Build history of the part. All positions in model axes, mm. A direction names the side the tool comes from. Give positions to 0.01 mm unless a question says otherwise; leave off trailing zeros. Loops run counter-clockwise (first coordinate to the right, second up) from the corner with the lowest first, then second, coordinate; pieces in that order, holes last. Notation, with made-up numbers: (-36.5, 19) -> (21.5, 19) arc R31 ccw to (21.5, 43) -> close; hole circle Ø9 at (-3.5, 47.5). An arc over 180 degrees is marked (long way). Answer in a Markdown table with one row per item. Add a question column.
from build123d import *

# Parameters (mm, degrees)
F2_DEPTH = 2.2225
F3_DEPTH = 12.7
F4_T     = -2.54


with BuildPart() as f2:
    # F0 (on Front) → F2 (new body, symmetric)
    with BuildSketch(Plane.XZ):
        with BuildLine():
            Line((40.6019, 72.8091), (-40.6019, 72.8091))
            ThreePointArc((-40.6019, 72.8091), (-43.295977, 71.693177), (-44.4119, 68.9991))
            Line((-44.4119, 68.9991), (-44.4119, -68.9991))
            ThreePointArc((-44.4119, -68.9991), (-43.295977, -71.693177), (-40.6019, -72.8091))
            Line((-40.6019, -72.8091), (40.6019, -72.8091))
            ThreePointArc((40.6019, -72.8091), (43.295977, -71.693177), (44.4119, -68.9991))
            Line((44.4119, -68.9991), (44.4119, 68.9991))
            ThreePointArc((44.4119, 68.9991), (43.295977, 71.693177), (40.6019, 72.8091))
        make_face()
    extrude(amount=F2_DEPTH, both=True)

    # F1 (on face) → F3 (cut, symmetric)
    with BuildSketch(Plane.XZ):
        with BuildLine():
            Line((15.494, -23.90966), (-15.494, -23.90966))
            ThreePointArc((-15.494, -23.90966), (-17.739064, -24.839596), (-18.669, -27.08466))
            Line((-18.669, -27.08466), (-18.669, -58.07266))
            ThreePointArc((-18.669, -58.07266), (-17.739064, -60.317724), (-15.494, -61.24766))
            Line((-15.494, -61.24766), (15.494, -61.24766))
            ThreePointArc((15.494, -61.24766), (17.739064, -60.317724), (18.669, -58.07266))
            Line((18.669, -58.07266), (18.669, -27.08466))
            ThreePointArc((18.669, -27.08466), (17.739064, -24.839596), (15.494, -23.90966))
        make_face()
    extrude(amount=F3_DEPTH, both=True, mode=Mode.SUBTRACT)

    # F4
    f4_openings = [f2.faces().sort_by_distance(p)[0] for p in [
        (0, 2.2225, 5.113505),
    ]]
    offset(amount=F4_T, openings=f4_openings)


solid = f2.part
(1) Saw through at B-B, the plane z = -40.5. List the corners of the cut face in (x, y), then the cut area to 3 significant figures.
(2) 3-axis set-ups, long thin cutter, end or side, ignore diameter. For faces 4 (the flat face through (-1, 0.317, 17)), 5 (the flat face through (18.669, 0, -43)), 6 (the cylindrical face through (-43.33, -0.03, -71.66)): which of +Z, -Z, +X, -X, +Y, -Y reach the whole face in a straight line?
(3) Saw through at C-C, the plane y = -1.55. List the corners of the cut face in (x, z) (3 decimals), then the cut area to 3 significant figures.
(4) Wall check: line 1 along Z through (x, y) = (3, 2); line 2 along X through (y, z) = (1.5, -64); line 3 along Z through (x, y) = (25.5, 1.2). Give the ranges that are in metal, low to high. Write a range as from..to.
(5) Flat gauge pin, fed straight in: pin 1 Ø3 at (x, z) = (23, -43.5) entering from +Y. Where does the tip first touch, or does it go through?
(6) Saw through at D-D, the plane x = -26. List the corners of the cut face in (y, z), then the cut area to 3 significant figures.
(7) Two-plate mould, pull along X, no slides. Class faces 1 (the cylindrical face through (-17.764, -0.031, -60.293)), 2 (the flat face through (-19, 2.222, -42)), 3 (the flat face through (-44.412, 0, 1)): released by +X, released by -X, zero draft, split by the parting line, or undercut.
(8) Saw through at A-A, the plane x = 13.5. List the corners of the cut face in (y, z).
Worked answers:
| question | item | result |
|---|---|---|
| 1 | outline | (-44.41, -2.22) -> (-18.67, -2.22) -> (-18.67, 2.22) -> (-21.21, 2.22) -> (-21.21, 0.32) -> (-41.87, 0.32) -> (-41.87, 2.22) -> (-44.41, 2.22) -> close; (18.67, -2.22) -> (44.41, -2.22) -> (44.41, 2.22) -> (41.87, 2.22) -> (41.87, 0.32) -> (21.21, 0.32) -> (21.21, 2.22) -> (18.67, 2.22) -> close |
| 1 | area | 150 mm^2 |
| 2 | face 4 | +Y |
| 2 | face 5 | +Y, -Y |
| 2 | face 6 | -Z, -X, +Y, -Y |
| 3 | outline | (-44.412, -68.999) arc R3.81 ccw to (-40.602, -72.809) -> (40.602, -72.809) arc R3.81 ccw to (44.412, -68.999) -> (44.412, 68.999) arc R3.81 ccw to (40.602, 72.809) -> (-40.602, 72.809) arc R3.81 ccw to (-44.412, 68.999) -> close; hole (-18.669, -58.073) arc R3.175 ccw to (-15.494, -61.248) -> (15.494, -61.248) arc R3.175 ccw to (18.669, -58.073) -> (18.669, -27.085) arc R3.175 ccw to (15.494, -23.91) -> (-15.494, -23.91) arc R3.175 ccw to (-18.669, -27.085) -> close |
| 3 | area | 11,500 mm^2 |
| 4 | line 1 | -72.81..-70.27, -63.79..-61.25, -23.91..-21.37, 70.27..72.81 |
| 4 | line 2 | -44.41..-41.87, 41.87..44.41 |
| 4 | line 3 | -72.81..-70.27, 70.27..72.81 |
| 5 | pin 1 | y = 0.32 |
| 6 | outline | (-2.22, -72.81) -> (2.22, -72.81) -> (2.22, -70.27) -> (0.32, -70.27) -> (0.32, 70.27) -> (2.22, 70.27) -> (2.22, 72.81) -> (-2.22, 72.81) -> close |
| 6 | area | 380 mm^2 |
| 7 | face 1 | undercut |
| 7 | face 2 | zero draft |
| 7 | face 3 | released by -X |
| 8 | outline | (-2.22, -72.81) -> (2.22, -72.81) -> (2.22, -70.27) -> (0.32, -70.27) -> (0.32, -63.79) -> (2.22, -63.79) -> (2.22, -61.25) -> (-2.22, -61.25) -> close; (-2.22, -23.91) -> (2.22, -23.91) -> (2.22, -21.37) -> (0.32, -21.37) -> (0.32, 70.27) -> (2.22, 70.27) -> (2.22, 72.81) -> (-2.22, 72.81) -> close |
